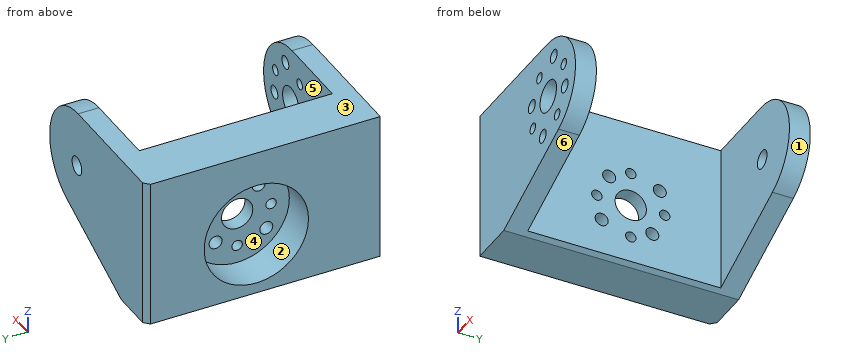
```python
from build123d import *

# Parameters (mm, degrees)
CYLINDER067_R                        = 1.75
CYLINDER067_DEPTH                    = 22
CYLINDER067_PITCH_ANGLE              = 90
CYLINDER061_R                        = 1.25
CYLINDER061_DEPTH                    = 22
CYLINDER061_PITCH_ANGLE              = 90
CYLINDER062_R                        = 1.25
CYLINDER062_DEPTH                    = 22
CYLINDER062_PITCH_ANGLE              = 90
CYLINDER060_R                        = 1.25
CYLINDER060_DEPTH                    = 22
CYLINDER060_PITCH_ANGLE              = 90
CYLINDER059_R                        = 1.25
CYLINDER059_DEPTH                    = 22
CYLINDER059_PITCH_ANGLE              = 90
CYLINDER065_R                        = 1.25
CYLINDER065_DEPTH                    = 22
CYLINDER065_PITCH_ANGLE              = 90
CYLINDER066_R                        = 1.25
CYLINDER066_DEPTH                    = 22
CYLINDER066_PITCH_ANGLE              = 90
CYLINDER064_R                        = 1.25
CYLINDER064_DEPTH                    = 22
CYLINDER064_PITCH_ANGLE              = 90
CYLINDER063_R                        = 1.25
CYLINDER063_DEPTH                    = 22
CYLINDER063_PITCH_ANGLE              = 90
FUSION047_ROLL_ANGLE                 = 34
FUSION047_PLACEMENT_ANGLE            = -90
CYLINDER058_R                        = 3
CYLINDER058_DEPTH                    = 22
CYLINDER058_PITCH_ANGLE              = 90
CYLINDER057_R                        = 3
CYLINDER057_DEPTH                    = 13
CYLINDER057_ROLL_ANGLE               = 90
CYLINDER056_R                        = 10
CYLINDER056_DEPTH                    = 10
CYLINDER056_ROLL_ANGLE               = 90
PAD007_DEPTH                         = 34
PAD005_DEPTH                         = 42
CHAMFER104_SIZE                      = 1
CLONE020_PLACEMENT_ANGLE             = -90
PART_MIRRORING007012_PLACEMENT_ANGLE = 180
BOX071_W                             = 47
BOX071_H                             = 42
BOX071_DEPTH                         = 35
BOX072_W                             = 47
BOX072_H                             = 42
BOX072_DEPTH                         = 35
SKETCH022_R                          = 1
POCKET018_DEPTH                      = 3
SKETCH023_R                          = 1
POCKET019_DEPTH                      = 4


with BuildPart() as cilindro011:
    # Cylinder067 → Cylinder067 (new body)
    with BuildSketch(Plane.XY):
        Circle(CYLINDER067_R)
    extrude(amount=CYLINDER067_DEPTH)


with BuildPart() as cilindro011_1:
    # Cylinder067 pitch: moved
    add(cilindro011.part.rotate(Axis((0, 0, 0), (0, 1, 0)), CYLINDER067_PITCH_ANGLE))


with BuildPart() as cilindro011_2:
    # Cylinder067 placement: moved
    add(cilindro011_1.part.moved(Location((-4.75, -32, 125.75))))


with BuildPart() as cilindro005:
    # Cylinder061 → Cylinder061 (new body)
    with BuildSketch(Plane.XY):
        Circle(CYLINDER061_R)
    extrude(amount=CYLINDER061_DEPTH)


with BuildPart() as cilindro005_1:
    # Cylinder061 pitch: moved
    add(cilindro005.part.rotate(Axis((0, 0, 0), (0, 1, 0)), CYLINDER061_PITCH_ANGLE))


with BuildPart() as cilindro005_2:
    # Cylinder061 placement: moved
    add(cilindro005_1.part.moved(Location((20.25, -38, 124.25))))


with BuildPart() as cilindro006:
    # Cylinder062 → Cylinder062 (new body)
    with BuildSketch(Plane.XY):
        Circle(CYLINDER062_R)
    extrude(amount=CYLINDER062_DEPTH)


with BuildPart() as cilindro006_1:
    # Cylinder062 pitch: moved
    add(cilindro006.part.rotate(Axis((0, 0, 0), (0, 1, 0)), CYLINDER062_PITCH_ANGLE))


with BuildPart() as cilindro006_2:
    # Cylinder062 placement: moved
    add(cilindro006_1.part.moved(Location((20.25, -26, 127.25))))


with BuildPart() as cilindro004:
    # Cylinder060 → Cylinder060 (new body)
    with BuildSketch(Plane.XY):
        Circle(CYLINDER060_R)
    extrude(amount=CYLINDER060_DEPTH)


with BuildPart() as cilindro004_1:
    # Cylinder060 pitch: moved
    add(cilindro004.part.rotate(Axis((0, 0, 0), (0, 1, 0)), CYLINDER060_PITCH_ANGLE))


with BuildPart() as cilindro004_2:
    # Cylinder060 placement: moved
    add(cilindro004_1.part.moved(Location((20.25, -30, 118.75))))


with BuildPart() as fusion046:
    # Cylinder059 → Cylinder059 (new body)
    with BuildSketch(Plane.XY):
        Circle(CYLINDER059_R)
    extrude(amount=CYLINDER059_DEPTH)


with BuildPart() as fusion046_1:
    # Cylinder059 pitch: moved
    add(fusion046.part.rotate(Axis((0, 0, 0), (0, 1, 0)), CYLINDER059_PITCH_ANGLE))


with BuildPart() as fusion046_2:
    # Cylinder059 placement: moved
    add(fusion046_1.part.moved(Location((20.25, -34, 132.75))))

    # Fusion046: union Cilindro005, Cilindro006, Cilindro004
    add(cilindro005_2.part)
    add(cilindro006_2.part)
    add(cilindro004_2.part)


with BuildPart() as cilindro009:
    # Cylinder065 → Cylinder065 (new body)
    with BuildSketch(Plane.XY):
        Circle(CYLINDER065_R)
    extrude(amount=CYLINDER065_DEPTH)


with BuildPart() as cilindro009_1:
    # Cylinder065 pitch: moved
    add(cilindro009.part.rotate(Axis((0, 0, 0), (0, 1, 0)), CYLINDER065_PITCH_ANGLE))


with BuildPart() as cilindro009_2:
    # Cylinder065 placement: moved
    add(cilindro009_1.part.moved(Location((20.25, -38, 124.25))))


with BuildPart() as cilindro010:
    # Cylinder066 → Cylinder066 (new body)
    with BuildSketch(Plane.XY):
        Circle(CYLINDER066_R)
    extrude(amount=CYLINDER066_DEPTH)


with BuildPart() as cilindro010_1:
    # Cylinder066 pitch: moved
    add(cilindro010.part.rotate(Axis((0, 0, 0), (0, 1, 0)), CYLINDER066_PITCH_ANGLE))


with BuildPart() as cilindro010_2:
    # Cylinder066 placement: moved
    add(cilindro010_1.part.moved(Location((20.25, -26, 127.25))))


with BuildPart() as cilindro008:
    # Cylinder064 → Cylinder064 (new body)
    with BuildSketch(Plane.XY):
        Circle(CYLINDER064_R)
    extrude(amount=CYLINDER064_DEPTH)


with BuildPart() as cilindro008_1:
    # Cylinder064 pitch: moved
    add(cilindro008.part.rotate(Axis((0, 0, 0), (0, 1, 0)), CYLINDER064_PITCH_ANGLE))


with BuildPart() as cilindro008_2:
    # Cylinder064 placement: moved
    add(cilindro008_1.part.moved(Location((20.25, -30, 118.75))))


with BuildPart() as fusion047:
    # Cylinder063 → Cylinder063 (new body)
    with BuildSketch(Plane.XY):
        Circle(CYLINDER063_R)
    extrude(amount=CYLINDER063_DEPTH)


with BuildPart() as fusion047_1:
    # Cylinder063 pitch: moved
    add(fusion047.part.rotate(Axis((0, 0, 0), (0, 1, 0)), CYLINDER063_PITCH_ANGLE))


with BuildPart() as fusion047_2:
    # Cylinder063 placement: moved
    add(fusion047_1.part.moved(Location((20.25, -34, 132.75))))

    # Fusion047: union Cilindro009, Cilindro010, Cilindro008
    add(cilindro009_2.part)
    add(cilindro010_2.part)
    add(cilindro008_2.part)


with BuildPart() as fusion047_3:
    # Fusion047 roll: moved
    add(fusion047_2.part.rotate(Axis((0, 0, 0), (1, 0, 0)), FUSION047_ROLL_ANGLE))


with BuildPart() as fusion047_4:
    # Fusion047 placement: moved
    add(fusion047_3.part.moved(Location((114.107998, 21, 33.646227))).rotate(Axis((114.107998, 21, 33.646227), (0, 0, 1)), FUSION047_PLACEMENT_ANGLE))


with BuildPart() as cilindro002:
    # Cylinder058 → Cylinder058 (new body)
    with BuildSketch(Plane.XY):
        Circle(CYLINDER058_R)
    extrude(amount=CYLINDER058_DEPTH)


with BuildPart() as cilindro002_1:
    # Cylinder058 pitch: moved
    add(cilindro002.part.rotate(Axis((0, 0, 0), (0, 1, 0)), CYLINDER058_PITCH_ANGLE))


with BuildPart() as cilindro002_2:
    # Cylinder058 placement: moved
    add(cilindro002_1.part.moved(Location((20.25, -32, 125.75))))


with BuildPart() as cilindro001:
    # Cylinder057 → Cylinder057 (new body)
    with BuildSketch(Plane.XY):
        Circle(CYLINDER057_R)
    extrude(amount=CYLINDER057_DEPTH)


with BuildPart() as cilindro001_1:
    # Cylinder057 roll: moved
    add(cilindro001.part.rotate(Axis((0, 0, 0), (1, 0, 0)), CYLINDER057_ROLL_ANGLE))


with BuildPart() as cilindro001_2:
    # Cylinder057 placement: moved
    add(cilindro001_1.part.moved(Location((17.25, -6, 120))))


with BuildPart() as cilindro:
    # Cylinder056 → Cylinder056 (new body)
    with BuildSketch(Plane.XY):
        Circle(CYLINDER056_R)
    extrude(amount=CYLINDER056_DEPTH)


with BuildPart() as cilindro_1:
    # Cylinder056 roll: moved
    add(cilindro.part.rotate(Axis((0, 0, 0), (1, 0, 0)), CYLINDER056_ROLL_ANGLE))


with BuildPart() as cilindro_2:
    # Cylinder056 placement: moved
    add(cilindro_1.part.moved(Location((17.25, -4, 120))))


with BuildPart() as pad007:
    # Sketch012 → Pad007 (new body)
    with BuildSketch(Plane(origin=(3, -12, -1), x_dir=(0, 1, 0), z_dir=(1, 0, 0))):
        Polygon((-4.882067, 101.940956), (-4.882067, 138.559921), (-40.571098, 142.373672), (-40.571098, 120.688431), align=None)
    extrude(amount=PAD007_DEPTH)


with BuildPart() as right_shoulder:
    # Sketch010 → Pad005 (new body)
    with BuildSketch(Plane.YZ.offset(-1)):
        with BuildLine():
            Line((-35.729516, 116.76657), (-15.773906, 107.988197))
            Line((-15.773906, 107.988197), (-7.000344, 107.988197))
            Line((-7.000344, 107.988197), (-7.000344, 136.642965))
            Line((-7.000344, 136.642965), (-31.550963, 136.642965))
            ThreePointArc((-31.550963, 136.642965), (-41.706398, 128.400491), (-35.729516, 116.76657))
        make_face()
    extrude(amount=PAD005_DEPTH)

    # Cut085: cut Pad007
    add(pad007.part, mode=Mode.SUBTRACT)

    # Cut086: cut Cilindro
    add(cilindro_2.part, mode=Mode.SUBTRACT)

    # Cut087: cut Cilindro001
    add(cilindro001_2.part, mode=Mode.SUBTRACT)

    # Chamfer104
    chamfer104_edges = [right_shoulder.edges().sort_by_distance(p)[0] for p in [
        (-1, -7.000344, 122.315581),
    ]]
    chamfer(chamfer104_edges, length=CHAMFER104_SIZE)

    # Cut088: cut Cilindro002
    add(cilindro002_2.part, mode=Mode.SUBTRACT)

    # Cut089: cut Fusion047
    add(fusion047_4.part, mode=Mode.SUBTRACT)

    # Cut090: cut Fusion046
    add(fusion046_2.part, mode=Mode.SUBTRACT)

    # Cut091: cut Cilindro011
    add(cilindro011_2.part, mode=Mode.SUBTRACT)


with BuildPart() as right_shoulder_1:
    # Clone020 placement: moved
    add(right_shoulder.part.moved(Location((-275, 70, 2.5))).rotate(Axis((-275, 70, 2.5), (0, 0, 1)), CLONE020_PLACEMENT_ANGLE))


with BuildPart() as left_shoulder:
    # Part__Mirroring007012: instance of right-shoulder
    add(right_shoulder_1.part.mirror(Plane(origin=(0, 0, 0), x_dir=(1, 0, 0), z_dir=(0, 1, 0))))


with BuildPart() as left_shoulder_1:
    # Part__Mirroring007012 placement: moved
    add(left_shoulder.part.moved(Location((-478, 0, 0))).rotate(Axis((-478, 0, 0), (0, 0, 1)), PART_MIRRORING007012_PLACEMENT_ANGLE))


with BuildPart() as clone_of_left_shoulder001:
    # Clone029 base: copy of left-shoulder
    add(left_shoulder_1.part)


with BuildPart() as clone_of_left_shoulder001_1:
    # Clone029 placement: moved
    add(clone_of_left_shoulder001.part.moved(Location((0, 3, 0))))


with BuildPart() as common:
    # Box071 → Box071 (new body)
    with BuildSketch(Plane(origin=(-205.102, 65.2498, 108.143), x_dir=(1, 0, 0), z_dir=(0, 0, 1))):
        with Locations((23.5, 21)):
            Rectangle(BOX071_W, BOX071_H)
    extrude(amount=BOX071_DEPTH)

    # Common: intersect Clone of left-shoulder001
    add(clone_of_left_shoulder001_1.part, mode=Mode.INTERSECT)


with BuildPart() as clone_of_left_shoulder:
    # Clone028 base: copy of left-shoulder
    add(left_shoulder_1.part)


with BuildPart() as leftshoulder_large_more_holes:
    # Box072 → Box072 (new body)
    with BuildSketch(Plane(origin=(-205.102, 24.2498, 108.143), x_dir=(1, 0, 0), z_dir=(0, 0, 1))):
        with Locations((23.5, 21)):
            Rectangle(BOX072_W, BOX072_H)
    extrude(amount=BOX072_DEPTH)

    # Common001: intersect Clone of left-shoulder
    add(clone_of_left_shoulder.part, mode=Mode.INTERSECT)

    # Fusion067: union Common
    add(common.part)

    # Sketch022 → Pocket018 (cut)
    with BuildSketch(Plane.YZ.offset(-186.117933)):
        with Locations((52.75, 129)):
            Circle(SKETCH022_R)
        with Locations((59.25, 122.5)):
            Circle(SKETCH022_R)
        with Locations((52.75, 116)):
            Circle(SKETCH022_R)
        with Locations((46.25, 122.5)):
            Circle(SKETCH022_R)
    extrude(amount=-POCKET018_DEPTH, mode=Mode.SUBTRACT)

    # Sketch023 → Pocket019 (cut)
    with BuildSketch(Plane.XZ.offset(-29)):
        with Locations((-174.220298, 133.896209)):
            Circle(SKETCH023_R)
        with Locations((-165.353791, 131.470298)):
            Circle(SKETCH023_R)
        with Locations((-167.779702, 122.603791)):
            Circle(SKETCH023_R)
        with Locations((-176.646209, 125.029702)):
            Circle(SKETCH023_R)
    extrude(amount=-POCKET019_DEPTH, mode=Mode.SUBTRACT)


solid = leftshoulder_large_more_holes.part
```
Can you work these out from the model? Positions are in its coordinate system, mm. Face numbers are marked on the shaded views. A direction names the side the tool comes from. Coordinates: 2 decimals unless noted, no trailing zeros. Write each loop counter-clockwise with the first axis right and the second up, starting at its lowest first coordinate (ties: lowest second). Pieces come first, ordered by that corner, then holes. Notation, with made-up numbers: (84, -37) - (135, -37) arc R22 cw to (135, -2) - close; hole circle Ø5 at (9.25, -9.5). An arc over 180 degrees is marked (long way). Return JSON: item names as keys, results as strings.
Q1. Thinking about a two-plate mould opening in Z: for the marked faces 1, 2 and 3, which applies, +Z half, -Z half, draft (parallel to the pull), parting line (faces both ways), or undercut?
Computed values:
{"face 1": "parting line", "face 2": "undercut", "face 3": "+Z half"}
Q2. If we section it at A-A (x = -193): Please give me the cut outline in (y, z).
Computed values:
{"outline": "(29, 110.49) - (74, 110.49) - (74, 139.14) - (29, 139.14) - close; hole circle Ø20 at (52.75, 122.5)"}
Q3. Please list where these lines run through material, in increasing order: L1, parallel to Y at x = -186.9, z = 122.5; L2, parallel to Y at x = -176, z = 116.25; L3, parallel to Z at x = -173, y = 31. Write a range as from..to.
Computed values:
{"L1": "y = 29..45.25, 47.25..49.75, 55.75..58.25, 60.25..74", "L2": "y = 29..33, 70..74", "L3": "z = 116.75..120, 122.5..126.01, 130.49..139.14"}
Q4. If we section it at C-C (x = -165): Please give me the cut outline in (y, z).
Computed values:
{"outline": "(29, 120.64) - (33, 120.64) - (33, 125.5) - (29, 125.5) - close; (29, 128) - (33, 128) - (33, 130.53) - (29, 130.53) - close; (29, 132.41) - (33, 132.41) - (33, 136.9) - (29, 136.9) - close; (70, 120.64) - (74, 120.64) - (74, 136.9) - (70, 136.9) - close"}
Q5. If we section it at B-B (y = 69): Please give me the cut outline in (x, z), then the cut area to 3 significant figures.
Computed values:
{"outline": "(-196, 110.49) - (-187.23, 110.49) - (-186.12, 110.98) - (-186.12, 139.14) - (-196, 139.14) - close", "area": "283 mm2"}
Q6. On a 3-axis mill with a long thin cutter (end or side, diameter ignored), from which of +Z, -Z, +X, -X, +Y, -Y can I reach the whole of each face in a straight line? I mean the marked faces 4, 5 and 6. Say none if no direction works.
Computed values:
{"face 4": "-X", "face 5": "+Z, -Z, +X", "face 6": "-Z, +X, +Y, -Y"}
Q7. I'm going to push flat-ended pins straight in: pin 1 Ø4 at (y, z) = (48.6, 127.1) entering from -X; pin 2 Ø1.6 at (x, z) = (-167.78, 122.6) entering from -Y; pin 3 Ø8 at (x, y) = (-171, 69) entering from -Z. Where does each tip first touch, or does it pass through?
Computed values:
{"pin 1": "stops at x = -189", "pin 2": "stops at y = 70", "pin 3": "stops at z = 115.92"}
